CAD build for the part. Positions are in the model's coordinates, mm. Face numbers are marked on the shaded views. A direction names the side the tool comes from. Coordinates: 2 decimals unless noted, no trailing zeros. Loops run counter-clockwise (first coordinate to the right, second up) from the corner with the lowest first, then second, coordinate; pieces in that order, holes last. Notation, with made-up numbers: M 80,-1 L 95,-1 A34 ccw 95,30 Z; hole C -38.5,17.5 d8. An arc over 180 degrees is marked long. Answer as a JSON object with one key per item and string values. Group by question number.
Autodesk Inventor part; units mm, degrees
ref_plane "YZ Plane" through (0, 0, 0) normal (1, 0, 0) x (0, 1, 0)
ref_plane "XZ Plane" through (0, 0, 0) normal (0, 1, 0) x (-1, 0, 0)
ref_plane "XY Plane" through (0, 0, 0) normal (0, 0, 1) x (1, 0, 0)
sketch "Sketch1" plane through (0, 0, 0) normal (1, 0, 0) x (0, 1, 0)
  line L0 (52.4, 0) -> (4, 0)
  line L1 (0, -4) -> (0, -52.4)
  line L2 (4, -56.4) -> (52.4, -56.4)
  line L3 (56.4, -52.4) -> (56.4, -4)
  line L4 (51.77, -4.63) -> (4.63, -4.63) construction
  line L5 (4.63, -4.63) -> (4.63, -51.77) construction
  line L6 (4.63, -51.77) -> (51.77, -51.77) construction
  line L7 (51.77, -51.77) -> (51.77, -4.63) construction
  circle A0 centre (51.77, -4.63) radius 2.5
  circle A1 centre (51.77, -51.77) radius 2.5
  circle A2 centre (4.63, -4.63) radius 2.5
  circle A3 centre (4.63, -51.77) radius 2.5
  arc A4 (56.4, -4) -> (52.4, 0) centre (52.4, -4) ccw
  arc A5 (52.4, -56.4) -> (56.4, -52.4) centre (52.4, -52.4) ccw
  arc A6 (0, -52.4) -> (4, -56.4) centre (4, -52.4) ccw
  arc A7 (4, 0) -> (0, -4) centre (4, -4) ccw
  point P0 (0, 0)
  point P1 (56.4, 0)
  point P2 (0, 0)
  point P3 (56.4, -56.4)
  point P4 (56.4, -28.2)
  point P5 (51.77, -28.2)
  point P6 (28.2, -51.77)
  point P7 (28.2, -56.4)
  dimension "d0" = 56.4
  dimension "d1" = 47.14
  dimension "d2" = 5
  dimension "d3" = 4
  dimension "d4" = 4
  dimension "d5" = 4
  dimension "d6" = 4
extrude "Extrusion1" add sketch "Sketch1" along normal blind 76
sketch "Sketch2" plane through (0, 0, 0) normal (-1, 0, 0) x (0, 0, 1)
  circle A0 centre (-28.2, 28.2) radius 19.05
  line L0 (-52.4, 56.4) -> (-4, 56.4)
  line L1 (-56.4, 4) -> (-56.4, 52.4)
  point P0 (0, 0)
  point P1 (-28.2, 56.4)
  point P2 (-56.4, 28.2)
  dimension "d9" = 38.1
extrude "Extrusion2" add sketch "Sketch2" along normal blind 1.6
sketch "Sketch3" plane through (-1.6, 28.2, -28.2) normal (-1, 0, 0) x (0, 0, 1)
  circle A0 centre (0, 0) radius 4
  circle A1 centre (0, 0) radius 19.05 construction
  point P0 (28.2, -28.2)
  dimension "d12" = 8
extrude "Extrusion3" add sketch "Sketch3" along normal blind 20
properties part number "Nema23"
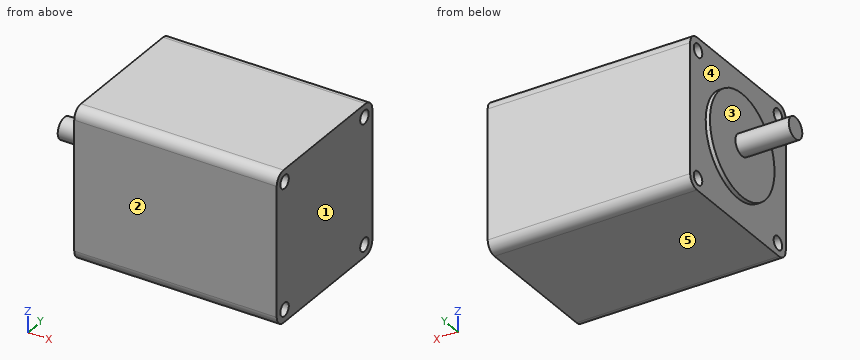
Item 1: Slice it at B-B, the plane z = -28.2. Write the cut outline in (x, y).
Item 2: Slice it at D-D, the plane y = 12. Write the cut outline in (x, z).
Item 3: Slice it at C-C, the plane y = 28.2. Write the cut outline in (x, z), then the cut area to 3 significant figures.
Item 4: Pull direction X, two halves, no side cores. Call the marked faces 1, 2 and 3: released by +X, released by -X, zero draft, split by the parting line, or undercut.
Item 5: Tool access for the marked faces 4 and 5: list every direction of +Z, -Z, +X, -X, +Y, -Y with a clear straight run to the whole face (end or side of a thin tool).
Item 6: Drill centre lines: L1, parallel to Z at x = 22, y = 4.63; L2, parallel to Y at x = 38, z = -51; L3, parallel to Y at x = 52, z = -54. Where is each one in solid material? Low to high. Write a range as from..to.
Item 7: Pin check, flat tips, straight feed: pin 1 (6 mm diameter, centred on y = 40, z = -27.5, fed in from -X); pin 2 (2 mm diameter, centred on y = 13, z = -48, fed in from -X). Stop position of each tip, or through.
Item 8: Slice it at A-A, the plane x = 39. Write the cut outline in (y, z), then the cut area to 3 significant figures.
Computed:
{
 "1": {"outline": "M -21.6,24.2 L -1.6,24.2 L -1.6,9.15 L 0,9.15 L 0,0 L 76,0 L 76,56.4 L 0,56.4 L 0,47.25 L -1.6,47.25 L -1.6,32.2 L -21.6,32.2 Z"},
 "2": {"outline": "M -1.6,-38.22 L 0,-38.22 L 0,-56.4 L 76,-56.4 L 76,0 L 0,0 L 0,-18.18 L -1.6,-18.18 Z"},
 "3": {"outline": "M -21.6,-32.2 L -1.6,-32.2 L -1.6,-47.25 L 0,-47.25 L 0,-56.4 L 76,-56.4 L 76,0 L 0,0 L 0,-9.15 L -1.6,-9.15 L -1.6,-24.2 L -21.6,-24.2 Z", "area": "4,510 mm2"},
 "4": {"face 1": "released by +X", "face 2": "zero draft", "face 3": "released by -X"},
 "5": {"face 4": "-X", "face 5": "-Z, +X, -X, +Y, -Y"},
 "6": {"L1": "-56.4..-54.27, -49.27..-7.13, -2.13..0", "L2": "0..2.25, 7.01..49.39, 54.15..56.4", "L3": "0.33..3.5, 5.76..50.64, 52.9..56.07"},
 "7": {"pin 1": "x = -1.6", "pin 2": "x = 0"},
 "8": {"outline": "M 0,-52.4 A4 ccw 4,-56.4 L 52.4,-56.4 A4 ccw 56.4,-52.4 L 56.4,-4 A4 ccw 52.4,0 L 4,0 A4 ccw 0,-4 Z; hole C 4.63,-51.77 d5; hole C 4.63,-4.63 d5; hole C 51.77,-51.77 d5; hole C 51.77,-4.63 d5", "area": "3,090 mm2"}
}
